Source: CAD feature listing. Evaluate the final solid. Frame: model axes, mm. A direction names the side the tool comes from. Coordinates: 2 decimals unless noted, no trailing zeros. Write each loop counter-clockwise with the first axis right and the second up, starting at its lowest first coordinate (ties: lowest second). Pieces come first, ordered by that corner, then holes. Notation, with made-up numbers: (35.5, 43.5) -> (49.5, 43.5) arc R12 cw to (49.5, 50.5) -> close; hole circle Ø7 at (15.25, 38.5). An arc over 180 degrees is marked (long way). One line per item, written item: value. Start each with the question number.
1. First-contact query: P1, Ø2, axis at x = 18.5, z = -10.5, coming from the +Y side; P2, Ø12, axis at y = 28, z = -1, coming from the +X side; P3, Ø11.5, axis at x = 22, y = 11, coming from the -Z side; P4, Ø1.4, axis at y = 37.5, z = 2.5, coming from the -X side. Flat tips, straight axial feed; report the tip coordinate or a pass-through.
2. Section query A-A, the plane x = 21. Output: boundary loops of the cut face in (y, z).
3. Mould query, pull axis Z, two halves, no side actions, for faces 5 (the flat face through (20, 38, 1)), 6 (the flat face through (5, -1, -14.95)), 7 (the cylindrical face through (20.28, -1.8, 1.83)), 8 (the flat face through (20, 0, -7)). Classes: released by +Z, released by -Z, zero draft, split by the parting line, or undercut.
4. Access query for faces 1 (the flat face through (34, -1, -14.95)), 2 (the flat face through (0.7, 35, 2)), 3 (the flat face through (8.8, 39, 2)), 4 (the flat face through (20, 15, 2.4)). Directions: +Z, -Z, +X, -X, +Y, -Y. A direction counts if a zero-diameter tool reaches every point of the face in a straight line with its end or side. Return the directions, or none.
5. Line query: line 1 (Z direction, x = 20, y = 17); line 2 (Y direction, x = 19, z = -6.75); line 3 (Z direction, x = 13.5, y = 35.5). Output: solid intervals per line, ascending.
6. Section query D-D, the plane x = 34. Output: boundary loops of the cut face in (y, z), and give its area (3 significant figures).
7. Section query B-B, the plane z = -5.5. Output: boundary loops of the cut face in (x, y).
8. Section query C-C, the plane y = 4. Output: boundary loops of the cut face in (x, z).
from build123d import *

# Parameters (mm, degrees)
SKETCH1_W                = 40
SKETCH1_H                = 40.6
BOSS_EXTRUDE1_DEPTH      = 2.4
SKETCH2_W                = 40
SKETCH2_H                = 2.4
BOSS_EXTRUDE2_DEPTH      = 17.35
SKETCH3_W                = 22.4
SKETCH3_H                = 2.6
CUT_EXTRUDE1_DEPTH       = 2.4
BOSS_EXTRUDE3_DEPTH      = 2.53
FILLET1_R                = 5.25
FILLET2_R                = 5.25
CUT_EXTRUDE2_DEPTH       = 16.4
FILLET3_R                = 2
CUT_EXTRUDE3_DEPTH       = 59.922512676
BOSS_EXTRUDE4_DEPTH      = 10
BOSS_EXTRUDE4_DEPTH_BACK = 10
FILLET4_R                = 0.05
CHAMFER1_SIZE            = 2
SKETCH9_W                = 0.7
SKETCH9_H                = 10
CUT_EXTRUDE4_DEPTH       = 60.009057176
FILLET5_R                = 2


with BuildPart() as part:
    # Sketch1 → Boss-Extrude1 (new body)
    with BuildSketch(Plane.XY):
        with Locations((20, 20.3)):
            Rectangle(SKETCH1_W, SKETCH1_H)
    extrude(amount=BOSS_EXTRUDE1_DEPTH)

    # Sketch2 → Boss-Extrude2 (add)
    with BuildSketch(Plane.XY.offset(2.4)):
        with Locations((20, -1.2)):
            Rectangle(SKETCH2_W, SKETCH2_H)
    extrude(amount=-BOSS_EXTRUDE2_DEPTH)

    # Sketch3 → Cut-Extrude1 (cut)
    with BuildSketch(Plane.XY.offset(2.4)):
        with Locations((20, 39.3)):
            Rectangle(SKETCH3_W, SKETCH3_H)
    extrude(amount=-CUT_EXTRUDE1_DEPTH, mode=Mode.SUBTRACT)

    # Sketch5 → Boss-Extrude3 (add)
    with BuildSketch(Plane.XY.offset(2.4)):
        Polygon((0, 40.6), (0, 34.6), (40, 34.6), (40, 40.6), (31.2, 40.6), (31.2, 38), (8.8, 38), (8.8, 40.6), align=None)
    extrude(amount=BOSS_EXTRUDE3_DEPTH)

    # Sketch4 → Cut-Revolve2 (revolve, cut)
    with BuildSketch(Plane(origin=(8.8, 0, 0), x_dir=(0, 0, -1), z_dir=(1, 0, 0))):
        with BuildLine():
            Line((-2.88, 39.3), (-4.58, 39.3))
            ThreePointArc((-4.58, 39.3), (-3.73, 38.45), (-2.88, 39.3))
        make_face()
    cut_revolve2 = revolve(axis=Axis((8.8, 39.3, 2.88), (0, 0, 1)), mode=Mode.SUBTRACT)

    # Mirror2: Cut-Revolve2 across plane
    add(cut_revolve2.mirror(Plane.ZY.offset(-20)), mode=Mode.SUBTRACT)

    # Fillet1
    fillet1_edges = [part.edges().sort_by_distance(p)[0] for p in [
        (0, 40.6, 2.465),
        (40, 40.6, 2.465),
    ]]
    fillet(fillet1_edges, radius=FILLET1_R)

    # Fillet2
    # the kernel refuses this fillet: 5.25 mm, written as the material it adds along each edge
    with BuildSketch(Plane(origin=(0, 34.6, 2.4), x_dir=(0, 0, 1), z_dir=(1, 0, 0))) as fillet2_piece_1:
        with BuildLine():
            CenterArc((5.25, 4.490445412), FILLET2_R, 180, 58.795429652)
            Line((0, 4.490445412), (-0.105, 4.490445412))
            Line((-0.105, 4.490445412), (-0.105, 0))
            Line((-0.105, 0), (0, -0.105))
            ThreePointArc((0, -0.105), (1.265, -0.105), (2.4756, -0.089808908))
            Line((2.4756, -0.089808908), (2.53, 0))
        make_face()
    extrude(amount=40)

    # Sketch6 → Cut-Extrude2 (cut)
    with BuildSketch(Plane.ZY.offset(-31.2)):
        Polygon((0, 40.6), (0, 38.6), (0.25, 40.6), align=None)
    cut_extrude2 = extrude(amount=-CUT_EXTRUDE2_DEPTH, mode=Mode.SUBTRACT)

    # Mirror3: Cut-Extrude2 across plane
    add(cut_extrude2.mirror(Plane.ZY.offset(-20)), mode=Mode.SUBTRACT)

    # Fillet3
    fillet3_edges = [part.edges().sort_by_distance(p)[0] for p in [
        (20, -2.4, 2.4),
    ]]
    fillet(fillet3_edges, radius=FILLET3_R)

    # Sketch7 → Cut-Extrude3 (cut, through all)
    with BuildSketch(Plane(origin=(0, 0, 0), x_dir=(1, 0, 0), z_dir=(0, 1, 0))):
        Polygon((37.6, 14.952), (40, 14), (40, 14.95), align=None)
    extrude(amount=-CUT_EXTRUDE3_DEPTH, mode=Mode.SUBTRACT)

    # Sketch8 → Boss-Extrude4 (add, two sides: drawn at the far end of the back side and taken through both)
    with BuildSketch(Plane.ZY.offset(-20).offset(-BOSS_EXTRUDE4_DEPTH_BACK)):
        Polygon((-14.95, 0), (-15.323046127, 0.8), (-14.95, -2.4), align=None)
    extrude(amount=BOSS_EXTRUDE4_DEPTH + BOSS_EXTRUDE4_DEPTH_BACK)

    # Fillet4
    fillet4_edges = [part.edges().sort_by_distance(p)[0] for p in [
        (20, 0.8, -15.323046127),
    ]]
    fillet(fillet4_edges, radius=FILLET4_R)

    # Chamfer1
    chamfer1_edges = [part.edges().sort_by_distance(p)[0] for p in [
        (20, 38, 4.93),
    ]]
    chamfer(chamfer1_edges, length=CHAMFER1_SIZE)

    # Sketch9 → Cut-Extrude4 (cut, through all)
    with BuildSketch(Plane(origin=(0, 0, 0), x_dir=(-1, 0, 0), z_dir=(0, 0, -1))):
        with Locations((-39.65, 35.6)):
            Rectangle(SKETCH9_W, SKETCH9_H)
        with Locations((-0.35, 35.6)):
            Rectangle(SKETCH9_W, SKETCH9_H)
    extrude(amount=-CUT_EXTRUDE4_DEPTH, mode=Mode.SUBTRACT)

    # Fillet5
    # the kernel refuses this fillet: 2 mm, written as the material it adds along each edge
    with BuildSketch(Plane(origin=(0.7, 30.6, 0), x_dir=(0, 1, 0), z_dir=(0, 0, 1))) as fillet5_piece_1_section:
        with BuildLine():
            CenterArc((1.519868415, 2), FILLET5_R, 220.541601874, 49.458398126)
            Line((0, 0.7), (-0.030397368, 0.674))
            ThreePointArc((-0.030397368, 0.674), (-0.04, 0.35), (-0.04, 0))
            Line((-0.04, 0), (0, -0.04))
            Line((0, -0.04), (1.519868415, -0.04))
            Line((1.519868415, -0.04), (1.519868415, 0))
        make_face()
    fillet5_piece_1 = extrude(amount=6.222629495, mode=Mode.PRIVATE)
    fillet5_piece_1 = fillet5_piece_1 - Plane(origin=(0.526032061, 30.109554588, 7.65), x_dir=(0, 0, 1), z_dir=(-1, 0, 0)) * Cylinder(5.25, 19, mode=Mode.PRIVATE)
    add(fillet5_piece_1)
    with BuildSketch(Plane(origin=(39.3, 30.6, 0), x_dir=(0, 1, 0), z_dir=(0, 0, 1))) as fillet5_piece_2_section:
        with BuildLine():
            CenterArc((1.519868415, -2), FILLET5_R, 90, 49.458398126)
            Line((0, -0.7), (-0.030397368, -0.674))
            ThreePointArc((-0.030397368, -0.674), (-0.04, -0.35), (-0.04, 0))
            Line((-0.04, 0), (0, 0.04))
            Line((0, 0.04), (1.519868415, 0.04))
            Line((1.519868415, 0.04), (1.519868415, 0))
        make_face()
    fillet5_piece_2 = extrude(amount=6.222629495, mode=Mode.PRIVATE)
    fillet5_piece_2 = fillet5_piece_2 - Plane(origin=(39.473967939, 30.109554588, 7.65), x_dir=(0, 0, 1), z_dir=(-1, 0, 0)) * Cylinder(5.25, 19, mode=Mode.PRIVATE)
    add(fillet5_piece_2)


solid = part.part
Computed values:
1. P1: stops at y = 0
1. P2: stops at x = 40
1. P3: stops at z = 0
1. P4: stops at x = 0.7
2. outline: (-2.4, -14.95) -> (0.49, -15.29) arc R0.05 ccw to (0.52, -15.19) -> (0, -14.95) -> (0, 0) -> (38, 0) -> (38, 2.93) -> (36, 4.93) -> (34.6, 4.93) arc R5.25 cw to (30.11, 2.4) -> (-0.4, 2.4) arc R2 ccw to (-2.4, 0.4) -> close
3. face 5: zero draft
3. face 6: released by -Z
3. face 7: released by +Z
3. face 8: undercut
4. face 1: -Z, +X, +Y, -Y
4. face 2: +Z, -Z, -X, +Y
4. face 3: +Z, +Y
4. face 4: +Z, +X, -X, -Y
5. line 1: z = 0 to 2.4
5. line 2: y = -2.4 to 0
5. line 3: z = 0 to 4.93
6. outline: (-2.4, -14.95) -> (0, -14.95) -> (0, 0) -> (38.6, 0) -> (40.6, 0.25) -> (40.6, 4.93) -> (34.6, 4.93) arc R5.25 cw to (30.11, 2.4) -> (-0.4, 2.4) arc R2 ccw to (-2.4, 0.4) -> close
6. area: 156 mm²
7. outline: (0, -2.4) -> (40, -2.4) -> (40, 0) -> (0, 0) -> close
8. outline: (0, 0) -> (40, 0) -> (40, 2.4) -> (0, 2.4) -> close
